Read the model definition and answer for the solid it produces. Units are mm, in the model's axes. Face numbers are marked on the shaded views. Round coordinates to 2 decimals unless told otherwise and drop trailing zeros. Order: outer loops, then holes, each group sorted by start corner. A loop starts at its lowest first (then second) coordinate and runs counter-clockwise, first axis right, second up. Notation, with made-up numbers: (30, -13.75) - (50, -13.75) arc R19 ccw to (50, 4.25) - close; hole circle Ø6 at (34.5, -2.75). An arc over 180 degrees is marked (long way). One line per question, with ' | ' between items. Start each with the question number.
1) Straight lines are drawn through the part: line 1 (Y direction, x = 0, z = -3.95); line 2 (Y direction, x = 0, z = 3.25). For each, find the intervals that lie inside material, in ascending order. Write a range as from..to.
2) The part is cut by section B-B, the plane z = 0. Give the vertices of the cut face in (x, y).
3) The part is cut by section A-A, the plane z = 4.5. Give the vertices of the cut face in (x, y).
4) The mould has two halves that part along X. Classify the marked faces 1, 2, 3 and 4: pulls with the +X half, pulls with the -X half, needs draft (parallel to the pull), parting line crosses it, or undercut.
5) Flat-ended cylindrical pins translate along their axes: pin 1 (9 mm diameter, centred on x = 0, y = 0, fed in from +Z); pin 2 (9.5 mm diameter, centred on x = 0, y = 0, fed in from +Z) (3 decimals); pin 3 (3 mm diameter, centred on x = -6, y = 1, fed in from +Z). Find the tip coordinate at first contact, or state that the pin passes through.
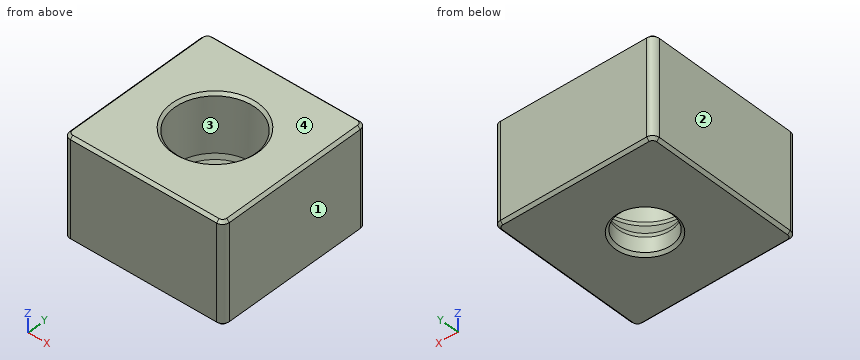
from build123d import *

# Parameters (mm, degrees)
SKETCH_W           = 23.7
SKETCH_H           = 23.7
PAD_DEPTH          = 15
FILLET003_R        = 1
CHAMFER002007_SIZE = 0.4


with BuildPart() as part:
    # Sketch → Pad (new body)
    with BuildSketch(Plane.XY):
        Rectangle(SKETCH_W, SKETCH_H)
    extrude(amount=PAD_DEPTH)

    # Fillet003
    fillet003_edges = [part.edges().sort_by_distance(p)[0] for p in [
        (-11.85, 11.85, 7.5),
        (-11.85, -11.85, 7.5),
        (11.85, 11.85, 7.5),
        (11.85, -11.85, 7.5),
    ]]
    fillet(fillet003_edges, radius=FILLET003_R)

    # Sketch001 → Groove (revolve, cut)
    with BuildSketch(Plane.XZ):
        Polygon((0, 0), (0, 15), (-6, 15), (-6, 6), (-4, 3), (-4, 0), align=None)
    revolve(axis=Axis((0, 0, 0), (0, 0, 1)), mode=Mode.SUBTRACT)

    # Chamfer002007
    chamfer002007_edges = [part.edges().sort_by_distance(p)[0] for p in [
        (0, 11.85, 15),
        (-11.557107, 11.557107, 15),
        (11.557107, 11.557107, 15),
        (-11.85, 0, 15),
        (11.85, 0, 15),
        (-11.557107, -11.557107, 15),
        (11.557107, -11.557107, 15),
        (0, -11.85, 15),
        (6, 0, 15),
        (0, 11.85, 0),
        (-11.557107, 11.557107, 0),
        (11.557107, 11.557107, 0),
        (-11.85, 0, 0),
        (11.85, 0, 0),
        (-11.557107, -11.557107, 0),
        (11.557107, -11.557107, 0),
        (0, -11.85, 0),
        (4, 0, 0),
        (4, 0, 3),
        (6, 0, 6),
    ]]
    chamfer(chamfer002007_edges, length=CHAMFER002007_SIZE)


with BuildPart() as part_1:
    # Body placement: moved
    add(part.part.moved(Location((0, 0, -5))))


solid = part_1.part
Values:
1) line 1: y = -11.85..-4, 4..11.85 | line 2: y = -11.85..-6, 6..11.85
2) outline: (-11.85, -10.85) arc R1 ccw to (-10.85, -11.85) - (10.85, -11.85) arc R1 ccw to (11.85, -10.85) - (11.85, 10.85) arc R1 ccw to (10.85, 11.85) - (-10.85, 11.85) arc R1 ccw to (-11.85, 10.85) - close; hole circle Ø10.67 at (0, 0)
3) outline: (-11.85, -10.85) arc R1 ccw to (-10.85, -11.85) - (10.85, -11.85) arc R1 ccw to (11.85, -10.85) - (11.85, 10.85) arc R1 ccw to (10.85, 11.85) - (-10.85, 11.85) arc R1 ccw to (-11.85, 10.85) - close; hole circle Ø12 at (0, 0)
4) face 1: pulls with the +X half | face 2: pulls with the -X half | face 3: undercut | face 4: needs draft
5) pin 1: stops at z = -1.25 | pin 2: stops at z = -0.875 | pin 3: stops at z = 10
